Input: part model. Units: mm. Frame: model coordinates. A direction names the side the tool comes from. Round coordinates to 2 decimals unless told otherwise and drop trailing zeros. Loops run counter-clockwise (first coordinate to the right, second up) from the corner with the lowest first, then second, coordinate; pieces in that order, holes last. Notation, with made-up numbers: (84, 20) -> (91, 20) arc R23 ccw to (91, 50) -> close; hole circle Ø7 at (23.25, 8). An arc over 180 degrees is marked (long way). Answer in a Markdown table with one row per item. Add a question column.
Q1. Mould query, pull axis X, two halves, no side actions, for faces 3 (the face through (0, 501, 50)), 4 (the face through (2032, 501, 50)), 5 (the face through (1422.4, 296, 52)), 6 (the face through (1002, 515, 101.6)). Classes: pulls with the +X half, pulls with the -X half, needs draft (parallel to the pull), parting line crosses it, or undercut.
Q2. Ray query, L1, parallel to X at y = 255, z = 84; L2, parallel to X at y = 605.5, z = 38; L3, parallel to Y at x = 1540, z = 40.5. Return the intervals inside material, ascending. Write a range as from..to.
Q3. Section C-C, the plane x = 1524. Output: boundary loops of the cut face in (y, z), and give its area (3 significant figures).
Q4. Section A-A, the plane y = 445.5. Output: boundary loops of the cut face in (x, z).
Q5. Section B-B, the plane z = 85. Output: boundary loops of the cut face in (x, y).
Q6. Reachability of faces 1 (the face through (1625.6, 288, 52)), 2 (the face through (1826, 0, 50)) from +Z, -Z, +X, -X, +Y, -Y: full face, straight path, thin tool, end or side. Return the list, or none.
```python
from build123d import *

# Parameters (mm, degrees)
F0_W     = 2032
F0_H     = 1016
F1_DEPTH = 101.6
F3_DEPTH = 101.601


with BuildPart() as f1:
    # F0 (on Top) → F1 (new body)
    with BuildSketch(Plane.XY):
        with Locations((1016, 508)):
            Rectangle(F0_W, F0_H)
    extrude(amount=F1_DEPTH)

    # F2 (on face) → F3 (cut, through all)
    with BuildSketch(Plane.XY.offset(101.6)):
        with BuildLine():
            Line((1422.4, 584.2), (1422.4, 0))
            Line((1422.4, 0), (1625.6, 0))
            Line((1625.6, 0), (1625.6, 584.2))
            ThreePointArc((1625.6, 584.2), (1524, 685.8), (1422.4, 584.2))
        make_face()
    extrude(amount=-F3_DEPTH, mode=Mode.SUBTRACT)


solid = f1.part
```
Answer block:
| question | item | result |
|---|---|---|
| 1 | face 3 | pulls with the -X half |
| 1 | face 4 | pulls with the +X half |
| 1 | face 5 | undercut |
| 1 | face 6 | needs draft |
| 2 | L1 | 0..1422.4, 1625.6..2032 |
| 2 | L2 | 0..1424.66, 1623.34..2032 |
| 2 | L3 | 684.53..1016 |
| 3 | outline | (685.8, 0) -> (1016, 0) -> (1016, 101.6) -> (685.8, 101.6) -> close |
| 3 | area | 33,500 mm^2 |
| 4 | outline | (0, 0) -> (1422.4, 0) -> (1422.4, 101.6) -> (0, 101.6) -> close; (1625.6, 0) -> (2032, 0) -> (2032, 101.6) -> (1625.6, 101.6) -> close |
| 5 | outline | (0, 0) -> (1422.4, 0) -> (1422.4, 584.2) arc R101.6 cw to (1625.6, 584.2) -> (1625.6, 0) -> (2032, 0) -> (2032, 1016) -> (0, 1016) -> close |
| 6 | face 1 | +Z, -Z, -Y |
| 6 | face 2 | +Z, -Z, +X, -X, -Y |
